Verification items for this drawing (mm, ordinates from the low corner). A direction names the side the tool comes from. Coordinates: 2 decimals unless noted, no trailing zeros. Write each loop counter-clockwise with the first axis right and the second up, starting at its lowest first coordinate (ties: lowest second). Pieces come first, ordered by that corner, then holes. Notation, with made-up numbers: (-5.75, 1) -> (22.25, 1) arc R26 ccw to (22.25, 27) -> close; hole circle Ø7 at (-23, 33). An arc over 180 degrees is marked (long way). Answer as CSV lines item,"result".
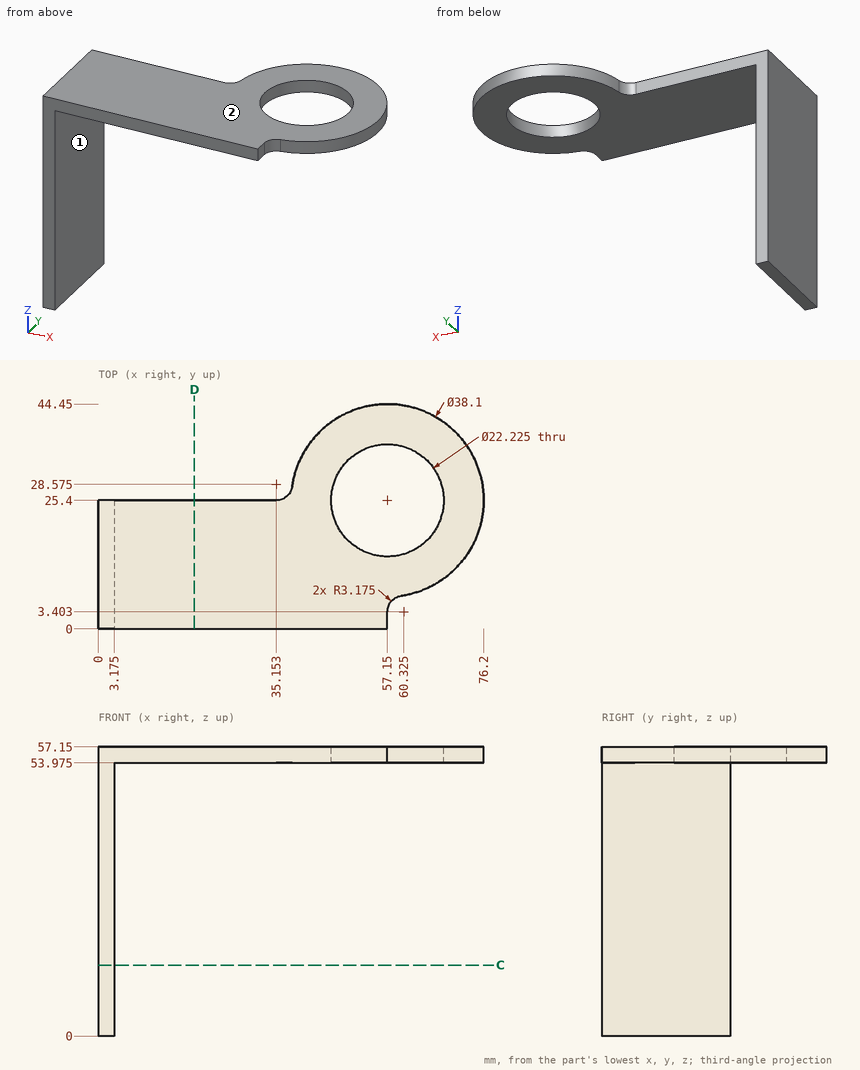
Item 1: Depth check by flat-ended pin: pin 1 Ø12 at (y, z) = (24.5, 37) entering from -X; pin 2 Ø3 at (x, y) = (37.5, 18) entering from -Z (3 decimals); pin 3 Ø1 at (y, z) = (2.5, 55) entering from +X; pin 4 Ø10 at (y, z) = (17.5, 46) entering from +X (3 decimals). Enter the tip coordinate at first touch or a pass-through.
Responses:
pin 1,"stops at x = 0"
pin 2,"stops at z = 53.975"
pin 3,"stops at x = 57.15"
pin 4,"stops at x = 3.175"
Item 2: Cross-section at D-D, the plane x = 19. Record the cut outline in (y, z) (3 decimals).
Responses:
outline,"(0, 53.975) -> (25.4, 53.975) -> (25.4, 57.15) -> (0, 57.15) -> close"
Item 3: Thickness scan on probe 1 along Y at (x, z) = (57, 56); probe 2 along Z at (x, y) = (41.5, 30) (3 decimals); probe 3 along X at (y, z) = (3.5, 43) (3 decimals). Record the ranges inside material, lowest first.
Responses:
probe 1,"y = 0 to 14.29, 36.51 to 44.45"
probe 2,"z = 53.975 to 57.15"
probe 3,"x = 0 to 3.175"
Item 4: Cross-section at C-C, the plane z = 14. Record the cut outline in (x, y) (3 decimals).
Responses:
outline,"(0, 0) -> (3.175, 0) -> (3.175, 25.4) -> (0, 25.4) -> close"
Item 5: Set-up check for the marked faces 1 and 2: record each of +Z, -Z, +X, -X, +Y, -Y from which the full face is reachable in a straight line by a thin tool's end or side.
Responses:
face 1,"-Z, +X, +Y, -Y"
face 2,"+Z, +X, -X, +Y, -Y"
